Design review of the part built by this model. Coordinates are the model's own, in mm. Face numbers are marked on the shaded views. Round coordinates to 2 decimals unless told otherwise and drop trailing zeros. Write each loop counter-clockwise with the first axis right and the second up, starting at its lowest first coordinate (ties: lowest second). Pieces come first, ordered by that corner, then holes.
from build123d import *

# Parameters (mm, degrees)
PAD016_DEPTH            = 24
POCKET028_DEPTH         = 5
SKETCH046_R             = 32
SKETCH046_R_2           = 6
POCKET029_DEPTH         = 24
BODY014_PLACEMENT_ANGLE = 180


with BuildPart() as part:
    # Sketch044 → Pad016 (new body)
    with BuildSketch(Plane.XY):
        with BuildLine():
            Line((5, 5), (119, 5))
            Line((119, 5), (119, 81))
            ThreePointArc((119, 81), (107.870058, 107.870058), (81, 119))
            Line((81, 119), (5, 119))
            Line((5, 119), (5, 5))
        make_face()
    extrude(amount=PAD016_DEPTH)

    # Sketch045 → Pocket028 (cut)
    with BuildSketch(Plane(origin=(0, 0, 0), x_dir=(1, 0, 0), z_dir=(0, 0, -1))):
        Polygon((12.374369, 12.374369), (123.206096, -98.457359), (98.457359, -123.206096), (-12.374369, -12.374369), (0, 0), align=None)
    extrude(amount=-POCKET028_DEPTH, mode=Mode.SUBTRACT)

    # Sketch046 → Pocket029 (cut)
    with BuildSketch(Plane.XY.offset(24)):
        Circle(SKETCH046_R)
        with Locations((85, 85)):
            Circle(SKETCH046_R_2)
    extrude(amount=-POCKET029_DEPTH, mode=Mode.SUBTRACT)


with BuildPart() as part_1:
    # Body014 placement: moved
    add(part.part.moved(Location((0, 210, -90))).rotate(Axis((0, 210, -90), (1, 0, 0)), BODY014_PLACEMENT_ANGLE))


solid = part_1.part
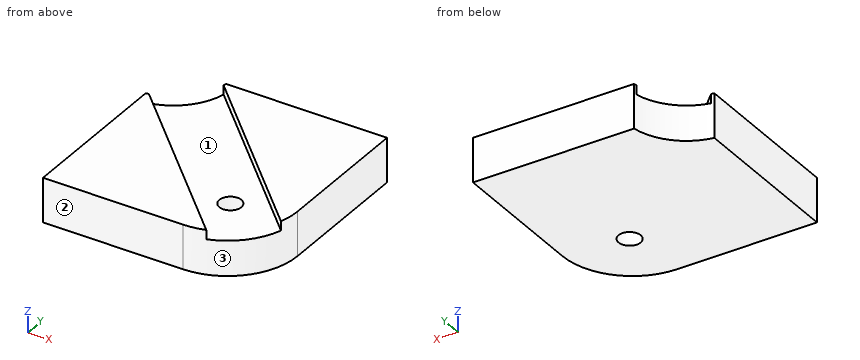
1) Add section A-A on z = -103.75. State the section outline as (x, y) points.
2) The part is to be moulded in two halves that separate along X. For the marked faces 1, 2 and 3, say which applies: pulls with the +X half, pulls with the -X half, needs draft (parallel to the pull), parting line crosses it, or undercut.
3) Add section C-C on y = 125. State the section outline as (x, z) points, and give its area (3 significant figures).
4) Add section B-B on x = 85. State the section outline as (y, z) points, and give its area (3 significant figures).
5) For line 1 along Y through (x, z) = (85, -109.5); line 2 along Z through (x, y) = (103.5, 130.5); line 3 along X through (y, z) = (119.5, -101.75), list the stretches that pass through material, from the lowest coordinate up.
6) Add section D-D on x = 54. State the section outline as (y, z) points.
7) For P1, Ø11, axis at x = 85, y = 125, coming from the +Z side; P2, Ø3, axis at y = 188.5, z = -96.5, coming from the -X side; P3, Ø1, axis at x = 105, z = -100.5, coming from the -Y side; P4, Ø2, axis at x = 28, z = -109, coming from the +Y side, all flat-tipped, find the tip position at first contact; note any pin that passes through.
Computed:
1. outline: (5, 91) - (81, 91) arc R38 ccw to (119, 129) - (119, 205) - (31.61, 205) arc R32 cw to (5, 178.39) - close; hole circle Ø12 at (85, 125)
2. face 1: undercut
2. face 2: needs draft
2. face 3: pulls with the +X half
3. outline: (5, -114) - (79, -114) - (79, -95) - (60.25, -95) - (60.25, -90) - (5, -90) - close; (91, -114) - (118.79, -114) - (118.79, -90) - (109.75, -90) - (109.75, -95) - (91, -95) - close
3. area: 2,260 mm2
4. outline: (91.21, -114) - (119, -114) - (119, -95) - (100.25, -95) - (100.25, -90) - (91.21, -90) - close; (131, -114) - (205, -114) - (205, -90) - (149.75, -90) - (149.75, -95) - (131, -95) - close
4. area: 2,260 mm2
5. line 1: y = 91.21 to 119, 131 to 205
5. line 2: z = -114 to -95
5. line 3: x = 5 to 82.6, 87.4 to 117.79
6. outline: (91, -114) - (205, -114) - (205, -90) - (180.75, -90) - (180.75, -95) - (131.25, -95) - (131.25, -90) - (91, -90) - close
7. P1: passes through
7. P2: stops at x = 22.25
7. P3: stops at y = 99.14
7. P4: stops at y = 196.47
